```python
from build123d import *

# Parameters (mm, degrees)
SKETCH1_R           = 38.1
BOSS_EXTRUDE1_DEPTH = 31.75
CHAMFER1_SIZE       = 1.524
SKETCH2_R           = 31.75
BOSS_EXTRUDE3_DEPTH = 4.7625
BOSS_EXTRUDE4_DEPTH = 9.525
SKETCH5_R           = 19.05
BOSS_EXTRUDE5_DEPTH = 12.7
BOSS_EXTRUDE6_DEPTH = 25.4
FILLET2_R           = 3.175


with BuildPart() as part:
    # Sketch1 → Boss-Extrude1 (new body)
    with BuildSketch(Plane(origin=(0, 0, 0), x_dir=(1, 0, 0), z_dir=(0, 1, 0))):
        with Locations(Location((0, 0, 0), (0, 0, 270))):
            Circle(SKETCH1_R)
    extrude(amount=-BOSS_EXTRUDE1_DEPTH)

    # Chamfer1
    chamfer1_edges = [part.edges().sort_by_distance(p)[0] for p in [
        (0, 0, -38.1),
    ]]
    chamfer(chamfer1_edges, length=CHAMFER1_SIZE)

    # Sketch2 → Boss-Extrude3 (add, symmetric)
    with BuildSketch(Plane(origin=(0, 0, 0), x_dir=(1, 0, 0), z_dir=(0, 1, 0))):
        with Locations(Location((0, 0, 0), (0, 0, 90))):
            Circle(SKETCH2_R)
    extrude(amount=BOSS_EXTRUDE3_DEPTH, both=True)

    # Sketch4 → Boss-Extrude4 (add)
    with BuildSketch(Plane(origin=(0, 0, 0), x_dir=(1, 0, 0), z_dir=(0, 1, 0))):
        Polygon((7.571021609, 26.429748164), (-13.335133431, 24.042174872), (-26.429748164, 7.571021609), (-24.042174872, -13.335133431), (-7.571021609, -26.429748164), (13.335133431, -24.042174872), (26.429748164, -7.571021609), (24.042174872, 13.335133431), align=None)
    extrude(amount=BOSS_EXTRUDE4_DEPTH)

    # Sketch5 → Boss-Extrude5 (add)
    with BuildSketch(Plane(origin=(0, 9.525, 0), x_dir=(1, 0, 0), z_dir=(0, 1, 0))):
        with Locations(Location((0, 0, 0), (0, 0, 270))):
            Circle(SKETCH5_R)
    extrude(amount=BOSS_EXTRUDE5_DEPTH)

    # Sketch6 → Boss-Extrude6 (add)
    with BuildSketch(Plane(origin=(0, 22.225, 0), x_dir=(1, 0, 0), z_dir=(0, 1, 0))):
        Polygon((4.716746996, 18.456836072), (-16.095939236, 10.189368975), (-14.664584525, -12.159459721), (7.032727569, -17.704328367), (19.011049196, 1.217583042), align=None)
    extrude(amount=BOSS_EXTRUDE6_DEPTH)

    # Fillet2
    fillet2_edges = [part.edges().sort_by_distance(p)[0] for p in [
        (0, 4.7625, 31.75),
    ]]
    fillet(fillet2_edges, radius=FILLET2_R)


solid = part.part
```
Here's how the part is built. I have some questions about the finished solid (model axes, mm). A direction names the side the tool comes from. Round coordinates to 2 decimals unless told otherwise and drop trailing zeros. Order: outer loops, then holes, each group sorted by start corner. A loop starts at its lowest first (then second) coordinate and runs counter-clockwise, first axis right, second up. Notation, with made-up numbers: (51.5, 7.25) -> (93.5, 7.25) arc R32 cw to (93.5, 40.25) -> close; hole circle Ø4 at (-33, 85). An arc over 180 degrees is marked (long way). Use a Markdown table: item, result. Add a question column.
(1) For faces 1 (the face through (13, 22.225, -11)), 2 (the face through (-8, 9.525, -18)), 3 (the face through (2.736, 7.11, 25.253)), which set-ups out of +Z, -Z, +X, -X, +Y, -Y let a thin tool reach every point of the face, with its end or its side?
(2) Suppose I cut it at A-A, the plane y = 33.5. Please give me the cut outline in (x, z).
(3) Suppose I cut it at D-D, the plane y = 19. Please give me the cut outline in (x, z).
(4) For pin 1 Ø1.5 at (y, z) = (-9, -20.5) entering from -X; pin 2 Ø10 at (x, y) = (-6, 23) entering from -Z; pin 3 Ø3 at (y, z) = (16, -13.5) entering from +X, each with a flat end and sliding along its axis, tell me the tip position at first contact or that it passes through.
(5) I need wall thicknesses on line 1 along Y through (x, z) = (-25.5, 19); line 2 along Y through (x, z) = (-19, 6.5) (3 decimals); line 3 along X through (y, z) = (-21.5, -33). Which ranges of each line are inside material? Lowest first, please.
Verdict:
| question | item | result |
|---|---|---|
| 1 | face 1 | -Z, +X, +Y |
| 1 | face 2 | +Y |
| 1 | face 3 | +Z, +X, +Y |
| 2 | outline | (-16.1, -10.19) -> (4.72, -18.46) -> (19.01, -1.22) -> (7.03, 17.7) -> (-14.66, 12.16) -> close |
| 3 | outline | circle Ø38.1 at (0, 0) |
| 4 | pin 1 | x = -32.58 |
| 4 | pin 2 | z = -19.02 |
| 4 | pin 3 | x = 14.8 |
| 5 | line 1 | -31.75 to 0 |
| 5 | line 2 | -31.75 to 9.525 |
| 5 | line 3 | -19.04 to 19.04 |
